CAD build for the part. Positions are in the model's coordinates, mm. A direction names the side the tool comes from. Give positions to 0.01 mm unless a question says otherwise; leave off trailing zeros. Loops run counter-clockwise (first coordinate to the right, second up) from the corner with the lowest first, then second, coordinate; pieces in that order, holes last. Notation, with made-up numbers: M 22.25,-25.75 L 32.25,-25.75 A15 ccw 32.25,-16.75 Z; hole C 49,-27.75 d11. An arc over 180 degrees is marked long. Answer as CSV lines item,"result".
```python
from build123d import *

# Parameters (mm, degrees)
SKETCH1_W                = 55
SKETCH1_H                = 25
BOSS_EXTRUDE1_DEPTH      = 4
SKETCH5_W                = 40.5
SKETCH5_H                = 17
CUT_EXTRUDE2_DEPTH       = 5
SKETCH6_W                = 55
SKETCH6_H                = 4.025345596
CUT_EXTRUDE3_DEPTH       = 5
SKETCH13_W               = 7.25
SKETCH13_H               = 20.974654404
BOSS_EXTRUDE3_DEPTH      = 8
SKETCH16_W               = 7.25
SKETCH16_H               = 20.974654404
BOSS_EXTRUDE4_DEPTH      = 8
SKETCH19_W               = 17
SKETCH19_H               = 4
BOSS_EXTRUDE5_DEPTH      = 4
SKETCH30_W               = 55
SKETCH30_H               = 4
BOSS_EXTRUDE6_DEPTH      = 7.5
SKETCH31_W               = 24.25
SKETCH31_H               = 4
BOSS_EXTRUDE7_DEPTH      = 7.5
SKETCH21_W               = 7.25
SKETCH21_H               = 16.974654404
CUT_EXTRUDE7_DEPTH       = 9
CUT_EXTRUDE9_DEPTH       = 56
CUT_EXTRUDE14_DEPTH      = 8.5
CUT_EXTRUDE14_DEPTH_BACK = 21.974654404


with BuildPart() as part:
    # Sketch1 → Boss-Extrude1 (new body)
    with BuildSketch(Plane(origin=(0, 0, 0), x_dir=(1, 0, 0), z_dir=(0, 1, 0))):
        Rectangle(SKETCH1_W, SKETCH1_H)
    extrude(amount=BOSS_EXTRUDE1_DEPTH)

    # Sketch5 → Cut-Extrude2 (cut, through all)
    with BuildSketch(Plane(origin=(0, 4, 0), x_dir=(1, 0, 0), z_dir=(0, 1, 0))):
        Rectangle(SKETCH5_W, SKETCH5_H)
    extrude(amount=-CUT_EXTRUDE2_DEPTH, mode=Mode.SUBTRACT)

    # Sketch6 → Cut-Extrude3 (cut, through all)
    with BuildSketch(Plane(origin=(0, 4, 0), x_dir=(1, 0, 0), z_dir=(0, 1, 0))):
        with Locations((0, 10.487327202)):
            Rectangle(SKETCH6_W, SKETCH6_H)
    extrude(amount=-CUT_EXTRUDE3_DEPTH, mode=Mode.SUBTRACT)

    # Sketch13 → Boss-Extrude3 (add)
    with BuildSketch(Plane(origin=(0, 4, 0), x_dir=(1, 0, 0), z_dir=(0, 1, 0))):
        with Locations((23.875, -2.012672798)):
            Rectangle(SKETCH13_W, SKETCH13_H)
    extrude(amount=-BOSS_EXTRUDE3_DEPTH)

    # Sketch16 → Boss-Extrude4 (add)
    with BuildSketch(Plane(origin=(0, 4, 0), x_dir=(1, 0, 0), z_dir=(0, 1, 0))):
        with Locations((-23.875, -2.012672798)):
            Rectangle(SKETCH16_W, SKETCH16_H)
    extrude(amount=-BOSS_EXTRUDE4_DEPTH)

    # Sketch19 → Boss-Extrude5 (add)
    with BuildSketch(Plane.XZ):
        with Locations((11.75, 10.5)):
            Rectangle(SKETCH19_W, SKETCH19_H)
    extrude(amount=BOSS_EXTRUDE5_DEPTH)

    # Sketch30 → Boss-Extrude6 (add)
    with BuildSketch(Plane.XY.offset(12.5)):
        with Locations((0, 2)):
            Rectangle(SKETCH30_W, SKETCH30_H)
    extrude(amount=BOSS_EXTRUDE6_DEPTH)

    # Sketch31 → Boss-Extrude7 (add)
    with BuildSketch(Plane.XY.offset(12.5)):
        with Locations((15.375, -2)):
            Rectangle(SKETCH31_W, SKETCH31_H)
    extrude(amount=BOSS_EXTRUDE7_DEPTH)

    # Sketch21 → Cut-Extrude7 (cut, through all)
    with BuildSketch(Plane(origin=(0, 4, 0), x_dir=(1, 0, 0), z_dir=(0, 1, 0))):
        with Locations((23.875, -0.012672798)):
            Rectangle(SKETCH21_W, SKETCH21_H)
    extrude(amount=-CUT_EXTRUDE7_DEPTH, mode=Mode.SUBTRACT)

    # Sketch25 → Cut-Extrude9 (cut, through all)
    with BuildSketch(Plane.ZY.offset(27.5)):
        with BuildLine():
            Line((2.314549123, -2), (-1.685450877, -2))
            ThreePointArc((-1.685450877, -2), (-3.685450877, 0), (-1.685450877, 2))
            Line((-1.685450877, 2), (2.314549123, 2))
            ThreePointArc((2.314549123, 2), (4.314549123, 0), (2.314549123, -2))
        make_face()
    extrude(amount=-CUT_EXTRUDE9_DEPTH, mode=Mode.SUBTRACT)

    # Sketch29 → Cut-Extrude14 (cut, two sides)
    with BuildSketch(Plane.XY.offset(12.5)) as cut_extrude14_sk:
        with BuildLine():
            Line((6.774762471, 2), (10.174762471, 2))
            ThreePointArc((10.174762471, 2), (12.174762471, 0), (10.174762471, -2))
            Line((10.174762471, -2), (6.774762471, -2))
            ThreePointArc((6.774762471, -2), (4.774762471, 0), (6.774762471, 2))
        make_face()
    extrude(amount=CUT_EXTRUDE14_DEPTH, mode=Mode.SUBTRACT)
    extrude(cut_extrude14_sk.sketch, amount=-CUT_EXTRUDE14_DEPTH_BACK, mode=Mode.SUBTRACT)


with BuildPart() as body_2:
    # Mirror1: mirrored copy
    add(part.part.mirror(Plane(origin=(27.5, 0, 14.25), x_dir=(0, 0, 1), z_dir=(1, 0, 0))))


solid = body_2.part
```
Q1. Cut at A-A (z = 13.5). Write the cut outline in (x, y).
Solution:
outline,"M 27.5,-4 L 51.75,-4 L 51.75,0 L 82.5,0 L 82.5,4 L 27.5,4 Z; hole M 44.83,-2 L 48.23,-2 A2 ccw 48.23,2 L 44.83,2 A2 ccw Z"
Q2. Pin check, flat tips, straight feed: P1, Ø1.2, axis at x = 79, y = -2.5, coming from the +Z side; P2, Ø6, axis at x = 61.5, z = 15.5, coming from the -Y side; P3, Ø2.5, axis at y = 0.5, z = 4.5, coming from the -X side; P4, Ø1, axis at y = 1, z = 1.5, coming from the +X side. Stop position of each tip, or through.
Solution:
P1,"stops at z = 12.5"
P2,"stops at y = 0"
P3,"stops at x = 75.25"
P4,"passes through"
Q3. Mould opens along Z. For faces 4 (the cylindrical face through (42.826, 0.044, 14.17)), 5 (the flat face through (46, 3, 8.5)), 6 (the cylindrical face through (78.926, -0.044, -3.685)), 7 (the flat face through (49, 3, 20)) say: released by +Z, released by -Z, zero draft, split by the parting line, or undercut.
Solution:
face 4,"zero draft"
face 5,"released by -Z"
face 6,"undercut"
face 7,"released by +Z"
Q4. Wall check: line 1 (Y direction, x = 77, z = 2.5); line 2 (Z direction, x = 41.5, y = -3.5); line 3 (X direction, y = 1.75, z = 7.25). Give the ranges that are in metal, low to high. Write a range as [from, to].
Solution:
line 1,"y = [-4, -1.99], [1.99, 4]"
line 2,"z = [8.5, 20]"
line 3,"x = [75.25, 82.5]"
Q5. Cut at D-D (z = 9.75). Write the cut outline in (x, y).
Solution:
outline,"M 27.5,-4 L 51.75,-4 L 51.75,0 L 75.25,0 L 75.25,-4 L 82.5,-4 L 82.5,4 L 27.5,4 Z; hole M 44.83,-2 L 48.23,-2 A2 ccw 48.23,2 L 44.83,2 A2 ccw Z"
Q6. Which spindle directions (+Z, -Z, +X, -X, +Y, -Y) get a long thin tool onto all of the face, cutting with end or side? Do faces 1 (the flat face through (75.25, -3, 2)), 2 (the flat face through (51.75, -2, 14)), 3 (the flat face through (79, -2, 0)). Say none if no direction does.
Solution:
face 1,"-Z, -Y"
face 2,"+Z, -Z, -Y"
face 3,"+X, -X"
Q7. Cut at B-B (y = 0.75). Write the cut outline in (x, z).
Solution:
outline,"M 27.5,8.5 L 42.97,8.5 L 42.97,20 L 27.5,20 Z; M 50.08,8.5 L 75.25,8.5 L 75.25,4.17 L 82.5,4.17 L 82.5,20 L 50.08,20 Z; M 75.25,-8.47 L 82.5,-8.47 L 82.5,-3.54 L 75.25,-3.54 Z"
Q8. Cut at C-C (x = 77). Write the cut outline in (y, z).
Solution:
outline,"M -4,-8.47 L 4,-8.47 L 4,20 L 0,20 L 0,12.5 L -4,12.5 Z; hole M -2,-1.69 A2 ccw 2,-1.69 L 2,2.31 A2 ccw -2,2.31 Z"
